from build123d import *

# Parameters (mm, degrees)
EXTRUDE_1_DEPTH     = 40
SKETCH_2_W          = 8
SKETCH_2_H          = 40
EXTRUDE_2_DEPTH     = 100
SKETCH_3_R          = 20
CUT_EXTRUDE_1_DEPTH = 149
SKETCH_4_W          = 49.783903804
SKETCH_4_H          = 113.982309312
CUT_EXTRUDE_3_DEPTH = 10
SKETCH_5_R          = 84.762192866
CUT_EXTRUDE_4_DEPTH = 20
SKETCH_6_W          = 140
SKETCH_6_H          = 20
EXTRUDE_3_DEPTH     = 8
SKETCH_7_R          = 10
EXTRUDE_4_DEPTH     = 60


with BuildPart() as part:
    # 草图1 → 凸台-拉伸1 (new body)
    with BuildSketch(Plane(origin=(0, 0, 0), x_dir=(1, 0, 0), z_dir=(0, 1, 0))):
        with BuildLine():
            Line((-74, 20), (-71.246052522, 20))
            ThreePointArc((-71.246052522, 20), (0, 74), (71.246052522, 20))
            Line((71.246052522, 20), (74, 20))
            Line((74, 20), (74, -20))
            Line((74, -20), (66, -20))
            Line((66, -20), (66, 0))
            ThreePointArc((66, 0), (0, 66), (-66, 0))
            Line((-66, 0), (-66, -20))
            Line((-66, -20), (-74, -20))
            Line((-74, -20), (-74, 20))
        make_face()
    extrude(amount=EXTRUDE_1_DEPTH)

    # 草图2 → 凸台-拉伸2 (add)
    with BuildSketch(Plane(origin=(0, 40, 0), x_dir=(1, 0, 0), z_dir=(0, 1, 0))):
        with Locations((-70, 0)):
            Rectangle(SKETCH_2_W, SKETCH_2_H)
        with Locations((70, 0)):
            Rectangle(SKETCH_2_W, SKETCH_2_H)
    extrude(amount=EXTRUDE_2_DEPTH)

    # 草图3 → 切除-拉伸1 (cut, through all)
    with BuildSketch(Plane.ZY.offset(74)):
        with Locations((0, 156)):
            Circle(SKETCH_3_R)
    extrude(amount=-CUT_EXTRUDE_1_DEPTH, mode=Mode.SUBTRACT)

    # 草图4 → 切除-拉伸3 (cut)
    with BuildSketch(Plane.ZY.offset(74)):
        with Locations((4.891951902, 96.991154656)):
            Rectangle(SKETCH_4_W, SKETCH_4_H)
    extrude(amount=-CUT_EXTRUDE_3_DEPTH, mode=Mode.SUBTRACT)

    # 草图5 → 切除-拉伸4 (cut)
    with BuildSketch(Plane.XZ):
        Circle(SKETCH_5_R)
        with BuildLine():
            Line((-71.246052522, 20), (-66, 20))
            Line((-66, 20), (-66, 0))
            Line((-66, 0), (-74, 0))
            ThreePointArc((-74, 0), (0, -74), (74, 0))
            Line((74, 0), (66, 0))
            Line((66, 0), (66, 20))
            Line((66, 20), (71.246052522, 20))
            ThreePointArc((71.246052522, 20), (0, 74), (-71.246052522, 20))
        make_face(mode=Mode.SUBTRACT)
    extrude(amount=-CUT_EXTRUDE_4_DEPTH, mode=Mode.SUBTRACT)

    # 草图6 → 凸台-拉伸3 (add)
    with BuildSketch(Plane(origin=(74, 0, 0), x_dir=(0, 0, -1), z_dir=(1, 0, 0))):
        with Locations((0, 50)):
            Rectangle(SKETCH_6_W, SKETCH_6_H)
    extrude(amount=-EXTRUDE_3_DEPTH)

    # 草图7 → 凸台-拉伸4 (add)
    with BuildSketch(Plane(origin=(74, 0, 0), x_dir=(0, 0, -1), z_dir=(1, 0, 0))):
        with Locations((-60, 50)):
            Circle(SKETCH_7_R)
        with Locations((60, 50)):
            Circle(SKETCH_7_R)
    extrude(amount=EXTRUDE_4_DEPTH)


solid = part.part
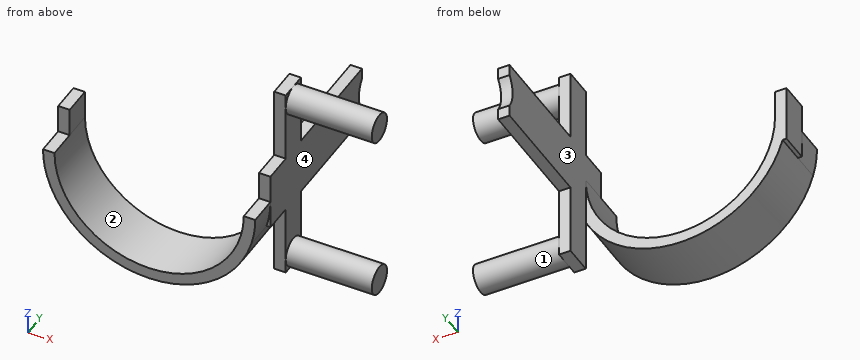
The listing builds one solid part. Answer for the finished solid, in the listing's coordinates (mm). Face numbers are marked on the shaded views. Round coordinates to 2 decimals unless told otherwise and drop trailing zeros. Write each loop counter-clockwise with the first axis right and the second up, starting at its lowest first coordinate (ties: lowest second). Pieces come first, ordered by that corner, then holes. Notation, with made-up numbers: (32, 49.5) - (88, 49.5) arc R32 ccw to (88, 84.5) - close; hole circle Ø10 at (60.5, 74.5). An arc over 180 degrees is marked (long way). Use a Markdown table: item, result. Add a question column.
1. The part is cut by section A-A (z = -6). Write down the section's boundary in (x, y).
2. The part is cut by section C-C (y = 16). Write down the section's boundary in (x, z).
3. Consider line 1 (X direction, y = 120.5, z = -14.5); line 2 (Y direction, x = 115.5, z = -59); line 3 (X direction, y = 13, z = -29.5). Determine where each line is inside the solid, lowest interval first.
4. Flat-ended cylindrical pins translate along their axes: P1, Ø1.4, axis at x = 73, y = 32, coming from the -Z side; P2, Ø9, axis at x = 71, z = 39.5, coming from the -Y side; P3, Ø1.4, axis at x = -72.5, z = -13.5, coming from the -Y side; P4, Ø6, axis at y = 26.5, z = 15, coming from the +X side. Find the tip coordinate at first contact, or state that the pin passes through.
5. The part is cut by section B-B (x = 95.5). Write down the section's boundary in (y, z).
6. The part is cut by section D-D (x = 0). Write down the section's boundary in (y, z).
7. For a pull along Z with two mould halves and no side action, classify the marked faces 1, 2, 3 and 4 as +Z half, -Z half, draft (parallel to the pull), parting line (faces both ways), or undercut.
Reported:
| question | item | result |
|---|---|---|
| 1 | outline | (-74, 20) - (-73.76, 20) - (-73.76, 0) - (-65.73, 0) - (-65.73, 40) - (-74, 40) - close; (65.73, 0) - (73.76, 0) - (73.76, 20) - (74, 20) - (74, 136.92) - (66, 136.92) - (66, 40) - (65.73, 40) - close |
| 2 | outline | (-74, 0) arc R74 ccw to (74, 0) - (66, 0) arc R66 cw to (-66, 0) - close |
| 3 | line 1 | 66 to 74 |
| 3 | line 2 | 40.05 to 59.95 |
| 3 | line 3 | -67.87 to -59.04, 59.04 to 67.87 |
| 4 | P1 | z = -20 |
| 4 | P2 | y = 40 |
| 4 | P3 | y = 0 |
| 4 | P4 | x = 74 |
| 5 | outline | circle Ø20 at (50, -60); circle Ø20 at (50, 60) |
| 6 | outline | (0, -74) - (40, -74) - (40, -66) - (0, -66) - close |
| 7 | face 1 | undercut |
| 7 | face 2 | +Z half |
| 7 | face 3 | draft |
| 7 | face 4 | undercut |
